Verification items for this drawing (mm, ordinates from the low corner). A direction names the side the tool comes from. Give positions to 0.01 mm unless a question says otherwise; leave off trailing zeros. Loops run counter-clockwise (first coordinate to the right, second up) from the corner with the lowest first, then second, coordinate; pieces in that order, holes last. Notation, with made-up numbers: (-21.5, 48) -> (8.5, 48) arc R10 ccw to (8.5, 61) -> close; hole circle Ø9 at (15, 31). An arc over 180 degrees is marked (long way). Write each question's results on one line, items separated by ' | '. Start each with the question number.
1) Scan lines: line 1 (Y direction, x = 38, z = 17.7); line 2 (Y direction, x = 7, z = 10); line 3 (Z direction, x = 14.5, y = 14). Record each from-to range of solid material in increasing order. Write a range as from..to.
2) Set-up check for the marked faces 1 and 2: record each of +Z, -Z, +X, -X, +Y, -Y from which the full face is reachable in a straight line by a thin tool's end or side.
3) Sectioned sample at B-B on x = 41. Record the cut outline in (y, z), then the cut area to 3 significant figures.
4) Depth check by flat-ended pin: pin 1 (1.5 mm diameter, centred on x = 12.5, z = 8, fed in from +Y); pin 2 (13 mm diameter, centred on x = 24.5, y = 33.5, fed in from -Z); pin 3 (2 mm diameter, centred on x = 37.3, y = 12, fed in from +Z); pin 4 (1.5 mm diameter, centred on y = 13, z = 6, fed in from -X). Enter the tip coordinate at first touch or a pass-through.
5) Sectioned sample at A-A on y = 44. Record the cut outline in (x, z).
6) Sectioned sample at C-C on z = 2.5. Record the cut outline in (x, y), then the cut area to 3 significant figures.
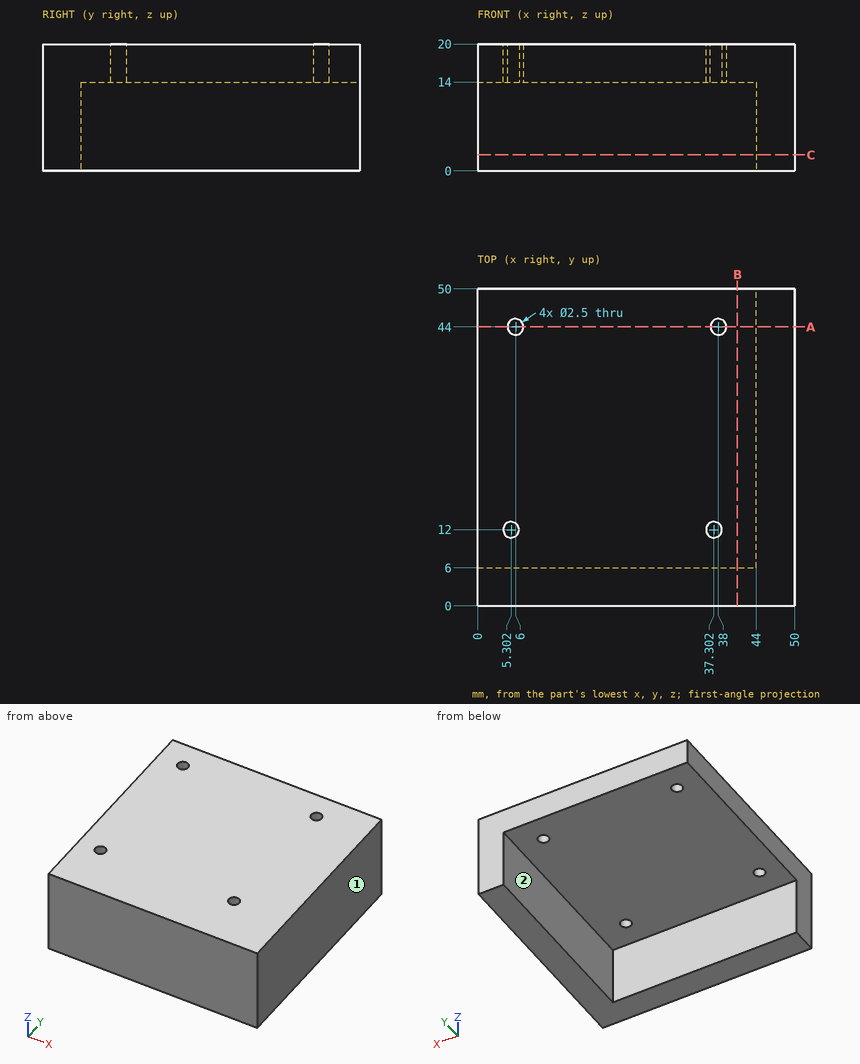
Result:
1) line 1: 0..10.96, 13.04..42.75, 45.25..50 | line 2: 0..6 | line 3: 14..20
2) face 1: +Z, -Z, +X, +Y, -Y | face 2: -Z, -X, +Y
3) outline: (0, 0) -> (6, 0) -> (6, 14) -> (50, 14) -> (50, 20) -> (0, 20) -> close | area: 384 mm^2
4) pin 1: y = 6 | pin 2: z = 14 | pin 3: through | pin 4: x = 44
5) outline: (0, 14) -> (4.75, 14) -> (4.75, 20) -> (0, 20) -> close; (7.25, 14) -> (36.75, 14) -> (36.75, 20) -> (7.25, 20) -> close; (39.25, 14) -> (44, 14) -> (44, 0) -> (50, 0) -> (50, 20) -> (39.25, 20) -> close
6) outline: (0, 0) -> (50, 0) -> (50, 50) -> (44, 50) -> (44, 6) -> (0, 6) -> close | area: 564 mm^2
